The drawing under review shows one solid part. Ordinate dimensions are in mm from its lowest x, y, z. Coordinates: 2 decimals unless noted, no trailing zeros. Order: outer loops, then holes, each group sorted by start corner. A loop starts at its lowest first (then second) coordinate and runs counter-clockwise, first axis right, second up. Notation, with made-up numbers: (-20.75, 73.25) -> (8.25, 73.25) arc R21 ccw to (8.25, 106.25) -> close; hole circle Ø5 at (-34, -19). An arc over 180 degrees is marked (long way). Use a Markdown table: item, result. Add a question column.
Q1. Wall thickness on probe 1 along X at (y, z) = (10, 3.3); probe 2 along Y at (x, z) = (40, 2.2); probe 3 along X at (y, z) = (41, 3.85): over which ranges is each line inside the solid? List them lowest first.
Q2. Insertion check: pin 1 (1.8 mm diameter, centred on x = 40, y = 10, fed in from -Z). The pin has a flat end and moves straight along its axis. Give the tip position at first contact, or say it passes through.
Q3. Add section A-A (x = 165). State the section outline as (y, z) points.
Q4. Add section C-C (z = 2.8). State the section outline as (x, y) points.
Q5. Add section B-B (y = 38.5). State the section outline as (x, z) points.
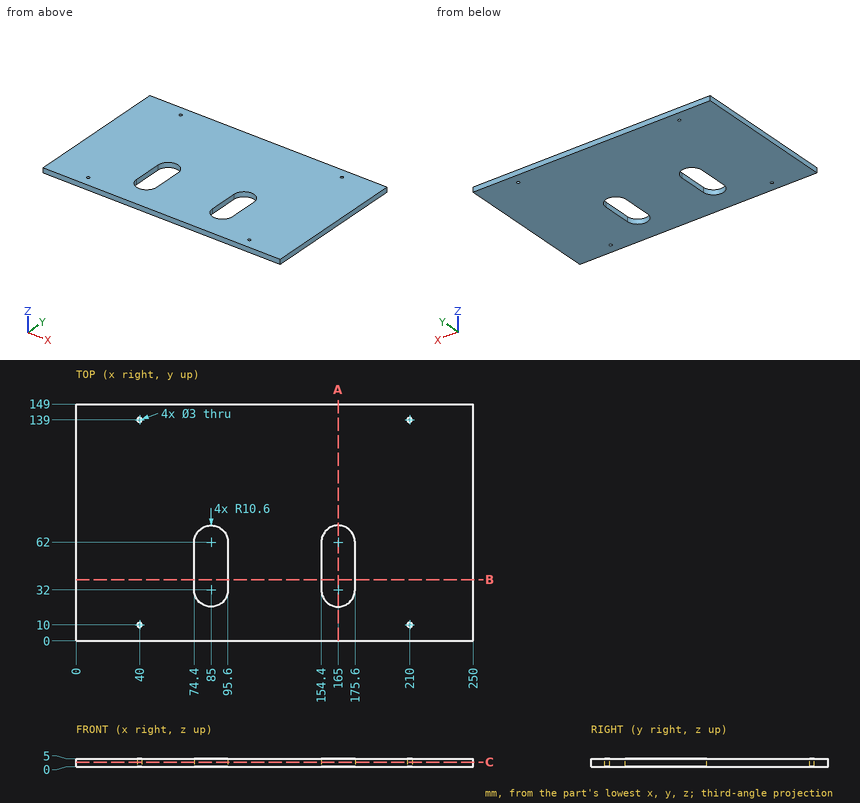
Established:
| question | item | result |
|---|---|---|
| 1 | probe 1 | 0 to 38.5, 41.5 to 208.5, 211.5 to 250 |
| 1 | probe 2 | 0 to 8.5, 11.5 to 137.5, 140.5 to 149 |
| 1 | probe 3 | 0 to 74.4, 95.6 to 154.4, 175.6 to 250 |
| 2 | pin 1 | through |
| 3 | outline | (0, 0) -> (21.4, 0) -> (21.4, 5) -> (0, 5) -> close; (72.6, 0) -> (149, 0) -> (149, 5) -> (72.6, 5) -> close |
| 4 | outline | (0, 0) -> (250, 0) -> (250, 149) -> (0, 149) -> close; hole circle Ø3 at (40, 10); hole circle Ø3 at (40, 139); hole (74.4, 32) arc R10.6 ccw to (95.6, 32) -> (95.6, 62) arc R10.6 ccw to (74.4, 62) -> close; hole (154.4, 32) arc R10.6 ccw to (175.6, 32) -> (175.6, 62) arc R10.6 ccw to (154.4, 62) -> close; hole circle Ø3 at (210, 10); hole circle Ø3 at (210, 139) |
| 5 | outline | (0, 0) -> (74.4, 0) -> (74.4, 5) -> (0, 5) -> close; (95.6, 0) -> (154.4, 0) -> (154.4, 5) -> (95.6, 5) -> close; (175.6, 0) -> (250, 0) -> (250, 5) -> (175.6, 5) -> close |
